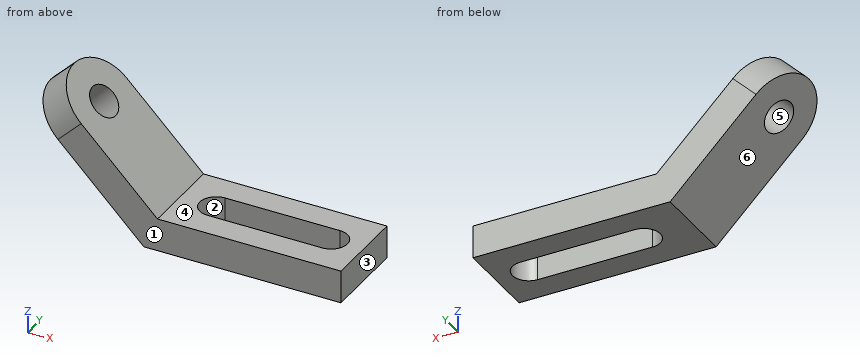
```python
from build123d import *

# Parameters (mm, degrees)
F1_DEPTH = 52
F2_R     = 10
F3_DEPTH = 144.8538137424
F5_DEPTH = 84.8538137424


with BuildPart() as f1:
    # F0 (on Front) → F1 (new body)
    with BuildSketch(Plane.XZ):
        Polygon((-130.7106781187, 60.7106781187), (-60, -10), (-60, 10), (-51.7157287525, 10), (-116.5685424949, 74.8528137424), align=None)
        Polygon((-60, -10), (60, -10), (60, 10), (-51.7157287525, 10), (-60, 10), align=None)
    extrude(amount=F1_DEPTH)

    # F2 (on face) → F3 (cut, through all)
    with BuildSketch(Plane(origin=(-35, 0, -35), x_dir=(0.7071067812, 0, -0.7071067812), z_dir=(-0.7071067812, 0, -0.7071067812))):
        with Locations((-109.3553390593, 26)):
            Circle(F2_R)
        with BuildLine():
            ThreePointArc((-135.3553390593, 26), (-127.7401153702, 44.3847763109), (-109.3553390593, 52))
            Line((-109.3553390593, 52), (-135.3553390593, 52))
            Line((-135.3553390593, 52), (-135.3553390593, 26))
        make_face()
        with BuildLine():
            Line((-135.3553390593, 0), (-109.3553390593, 0))
            ThreePointArc((-109.3553390593, 0), (-127.7401153702, 7.6152236891), (-135.3553390593, 26))
            Line((-135.3553390593, 26), (-135.3553390593, 0))
        make_face()
    extrude(amount=-F3_DEPTH, mode=Mode.SUBTRACT)

    # F4 (on face) → F5 (cut, through all)
    with BuildSketch(Plane(origin=(0, 0, -10), x_dir=(1, 0, 0), z_dir=(0, 0, -1))):
        with BuildLine():
            ThreePointArc((40, 16), (50, 26), (40, 36))
            Line((40, 36), (-30, 36))
            ThreePointArc((-30, 36), (-40, 26), (-30, 16))
            Line((-30, 16), (40, 16))
        make_face()
    extrude(amount=-F5_DEPTH, mode=Mode.SUBTRACT)


solid = f1.part
```
Model file for the job. Use its own axes, mm. Face numbers are marked on the shaded views. A direction names the side the tool comes from. Give positions to 0.01 mm unless a question says otherwise; leave off trailing zeros. Loops run counter-clockwise (first coordinate to the right, second up) from the corner with the lowest first, then second, coordinate; pieces in that order, holes last. Notation, with made-up numbers: (50, -30) -> (79, -30) arc R24 ccw to (79, -9) -> close; hole circle Ø4 at (-33, 69.25). An arc over 180 degrees is marked (long way). Use CSV: the item, a comma, the result in double quotes. Start each with the question number.
1) Slice it at D-D on y = -3.5. Give the cut face in (x, z).
2) Tool access for the marked faces 1 and 2: list every direction of +Z, -Z, +X, -X, +Y, -Y with a clear straight run to the whole face (end or side of a thin tool).
3) Slice it at B-B on x = 8.5. Give the cut face in (y, z).
4) Mould opens along X. For the marked faces 3, 4, 5 and 6 say: released by +X, released by -X, zero draft, split by the parting line, or undercut.
5) Slice it at C-C on y = -30. Give the cut face in (x, z).
6) Wall check: line 1 (Y direction, x = 36, z = -3); line 2 (Z direction, x = 11, y = -45.5); line 3 (X direction, y = -22, z = 3.5). Give the ranges that are in metal, low to high.
7) Flat gauge pins, fed straight in: pin 1 Ø5 at (y, z) = (-10.5, 30.5) entering from -X; pin 2 Ø22 at (x, z) = (15.5, -4) entering from +Y; pin 3 Ø12 at (x, y) = (-68.5, -41.5) entering from +Z; pin 4 Ø12 at (y, z) = (-33, 63) entering from +X. Where does each tip first touch, or does it go through?
8) Slice it at A-A on z = 1.5. Give the cut face in (x, y).
Computed values:
1,outline,"(-121.54, 51.54) -> (-60, -10) -> (60, -10) -> (60, 10) -> (-51.72, 10) -> (-107.4, 65.68) -> close"
2,face 1,"+Z, -Z, +X, -X, -Y"
2,face 2,"+Z, -Z"
3,outline,"(-52, -10) -> (-36, -10) -> (-36, 10) -> (-52, 10) -> close; (-16, -10) -> (0, -10) -> (0, 10) -> (-16, 10) -> close"
4,face 3,"released by +X"
4,face 4,"zero draft"
4,face 5,"undercut"
4,face 6,"released by -X"
5,outline,"(-130.49, 60.49) -> (-118.81, 48.81) -> (-104.66, 62.95) -> (-116.35, 74.63) -> close; (-105.85, 35.85) -> (-60, -10) -> (-39.17, -10) -> (-39.17, 10) -> (-51.72, 10) -> (-91.7, 49.99) -> close; (49.17, -10) -> (60, -10) -> (60, 10) -> (49.17, 10) -> close"
6,line 1,"y = -52 to -36, -16 to 0"
6,line 2,"z = -10 to 10"
6,line 3,"x = -73.5 to -39.17, 49.17 to 60"
7,pin 1,"stops at x = -103"
7,pin 2,"stops at y = 0"
7,pin 3,"stops at z = 32.78"
7,pin 4,"stops at x = -99.43"
8,outline,"(-71.5, -52) -> (60, -52) -> (60, 0) -> (-71.5, 0) -> close; hole (-30, -36) -> (40, -36) arc R10 ccw to (40, -16) -> (-30, -16) arc R10 ccw to start"
